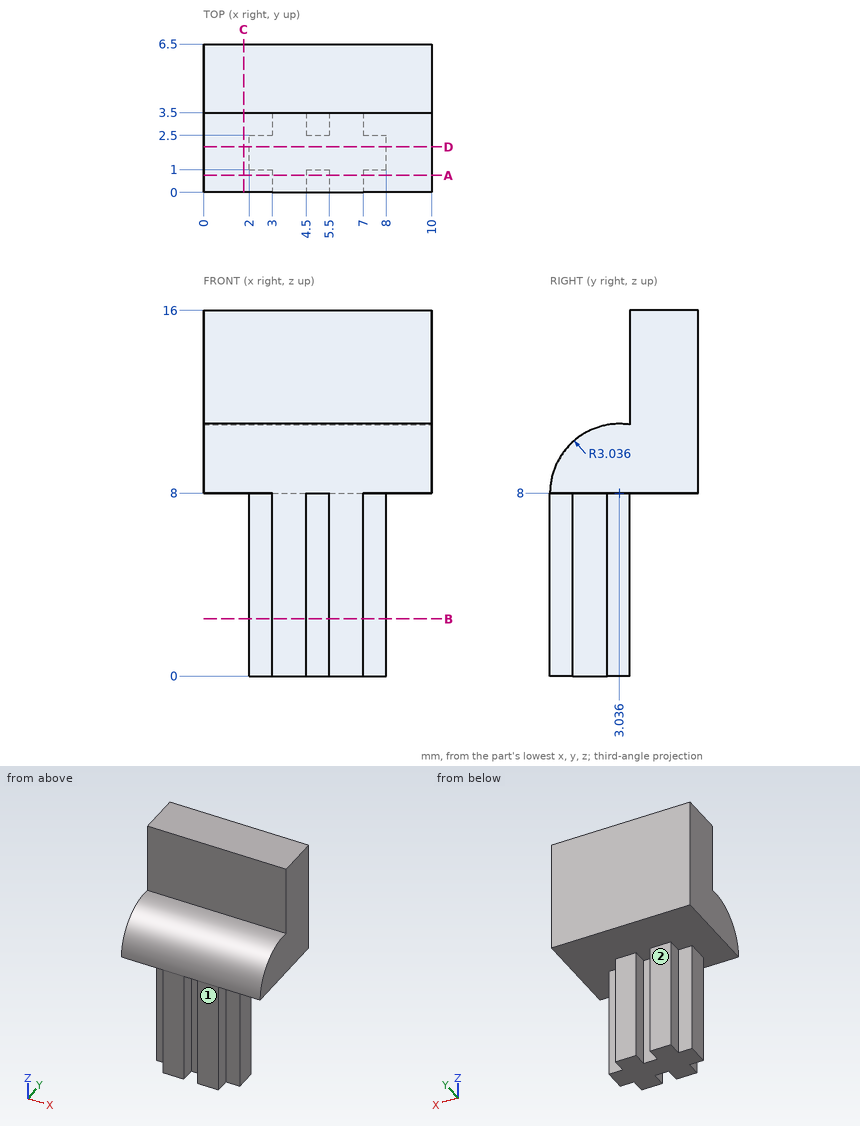
Could you check a few things on this drawing? It's one solid part, dimensions in mm from its lowest x, y, z. A direction names the side the tool comes from. Round coordinates to 2 decimals unless told otherwise and drop trailing zeros. Write each loop counter-clockwise with the first axis right and the second up, starting at its lowest first coordinate (ties: lowest second). Pieces come first, ordered by that corner, then holes. Notation, with made-up numbers: (-37.75, 7.5) -> (-26.75, 7.5) arc R23 cw to (-26.75, 43.5) -> close; hole circle Ø4 at (-26.5, 88). An arc over 180 degrees is marked (long way). Use one line per item in the form item = value. Start each with the question number.
Q1. Imagine slicing it at C-C (x = 1.75). Please give me the cut outline in (y, z).
Q2. I'm going to push flat-ended pins straight in: P1, Ø0.8, axis at x = 6.5, z = 5, coming from the +Y side; P2, Ø1.1, axis at y = 0.5, z = 2.5, coming from the +X side; P3, Ø0.8, axis at x = 2.5, z = 5.5, coming from the +Y side; P4, Ø1.1, axis at x = 5, z = 3, coming from the -Y side. Where does each tip first touch, or does it pass through?
Q3. Imagine slicing it at B-B (z = 2.5). Please give me the cut outline in (x, y), then the cut area to 3 significant figures.
Q4. Imagine slicing it at D-D (y = 2). Please give me the cut outline in (x, z).
Q5. If I drill on probe 1 along Y at (x, z) = (1.5, 11.25); probe 2 along Z at (x, y) = (3, 5.5); probe 3 along Y at (x, z) = (5.25, 4), over which ranges is the centre line in solid material (lowest first)? Write a range as [from, to].
Q6. Imagine slicing it at A-A (y = 0.75). Please give me the cut outline in (x, z).
Q7. Which directions (+Z, -Z, +X, -X, +Y, -Y) give clear straight access to the entire face, cutting with the end or side of a thin tool? Please do the marked faces 1 and 2.
Worked out:
q1.outline = (0, 8) -> (6.5, 8) -> (6.5, 16) -> (3.5, 16) -> (3.5, 11) arc R3.04 ccw to start
q2.P1 = 3.5
q2.P2 = 8
q2.P3 = 2.5
q2.P4 = 0
q3.outline = (2, 1) -> (3, 1) -> (3, 0) -> (4.5, 0) -> (4.5, 1) -> (5.5, 1) -> (5.5, 0) -> (7, 0) -> (7, 1) -> (8, 1) -> (8, 2.5) -> (7, 2.5) -> (7, 3.5) -> (5.5, 3.5) -> (5.5, 2.5) -> (4.5, 2.5) -> (4.5, 3.5) -> (3, 3.5) -> (3, 2.5) -> (2, 2.5) -> close
q3.area = 15.0 mm^2
q4.outline = (0, 8) -> (2, 8) -> (2, 0) -> (8, 0) -> (8, 8) -> (10, 8) -> (10, 10.85) -> (0, 10.85) -> close
q5.probe_1 = [3.5, 6.5]
q5.probe_2 = [8, 16]
q5.probe_3 = [1, 2.5]
q6.outline = (0, 8) -> (3, 8) -> (3, 0) -> (4.5, 0) -> (4.5, 8) -> (5.5, 8) -> (5.5, 0) -> (7, 0) -> (7, 8) -> (10, 8) -> (10, 10) -> (0, 10) -> close
q7.face_1 = +Z, -Z, +X, -X, -Y
q7.face_2 = -Z, +X, -X, +Y
